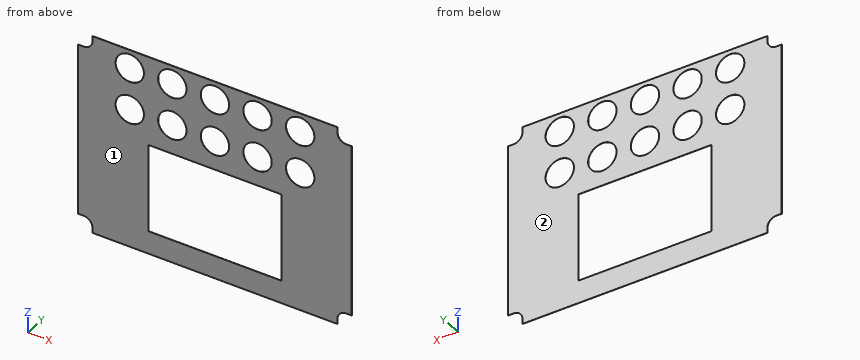
from build123d import *

# Parameters (mm, degrees)
SKETCH1_W           = 154
SKETCH1_H           = 114
BOSS_EXTRUDE1_DEPTH = 0.1
CUT_EXTRUDE1_DEPTH  = 3
SKETCH3_R           = 8
SKETCH3_W           = 75
SKETCH3_H           = 50
CUT_EXTRUDE2_DEPTH  = 1


with BuildPart() as part:
    # Sketch1 → Boss-Extrude1 (new body)
    with BuildSketch(Plane(origin=(0, 0, 0), x_dir=(1, 0, 0), z_dir=(0, 1, 0))):
        Rectangle(SKETCH1_W, SKETCH1_H)
    extrude(amount=BOSS_EXTRUDE1_DEPTH)

    # Sketch2 → Cut-Extrude1 (cut)
    with BuildSketch(Plane(origin=(0, 0.1, 0), x_dir=(1, 0, 0), z_dir=(0, 1, 0))):
        with BuildLine():
            Line((-52.05, -19.483379374), (-52.05, -25.516620626))
            ThreePointArc((-52.05, -25.516620626), (-48, -27.55), (-43.95, -25.516620626))
            Line((-43.95, -25.516620626), (-43.95, -19.483379374))
            ThreePointArc((-43.95, -19.483379374), (-48, -17.45), (-52.05, -19.483379374))
        make_face()
        with BuildLine():
            Line((-19.95, -19.483379374), (-19.95, -25.516620626))
            ThreePointArc((-19.95, -25.516620626), (-24, -27.55), (-28.05, -25.516620626))
            Line((-28.05, -25.516620626), (-28.05, -19.483379374))
            ThreePointArc((-28.05, -19.483379374), (-24, -17.45), (-19.95, -19.483379374))
        make_face()
        with BuildLine():
            Line((4.05, -19.483379374), (4.05, -25.516620626))
            ThreePointArc((4.05, -25.516620626), (0, -27.55), (-4.05, -25.516620626))
            Line((-4.05, -25.516620626), (-4.05, -19.483379374))
            ThreePointArc((-4.05, -19.483379374), (0, -17.45), (4.05, -19.483379374))
        make_face()
        with BuildLine():
            Line((28.05, -19.483379374), (28.05, -25.516620626))
            ThreePointArc((28.05, -25.516620626), (24, -27.55), (19.95, -25.516620626))
            Line((19.95, -25.516620626), (19.95, -19.483379374))
            ThreePointArc((19.95, -19.483379374), (24, -17.45), (28.05, -19.483379374))
        make_face()
        with BuildLine():
            Line((52.05, -19.483379374), (52.05, -25.516620626))
            ThreePointArc((52.05, -25.516620626), (48, -27.55), (43.95, -25.516620626))
            Line((43.95, -25.516620626), (43.95, -19.483379374))
            ThreePointArc((43.95, -19.483379374), (48, -17.45), (52.05, -19.483379374))
        make_face()
        with BuildLine():
            Line((-19.95, -43.483379374), (-19.95, -49.516620626))
            ThreePointArc((-19.95, -49.516620626), (-24, -51.55), (-28.05, -49.516620626))
            Line((-28.05, -49.516620626), (-28.05, -43.483379374))
            ThreePointArc((-28.05, -43.483379374), (-24, -41.45), (-19.95, -43.483379374))
        make_face()
        with BuildLine():
            Line((4.05, -43.483379374), (4.05, -49.516620626))
            ThreePointArc((4.05, -49.516620626), (0, -51.55), (-4.05, -49.516620626))
            Line((-4.05, -49.516620626), (-4.05, -43.483379374))
            ThreePointArc((-4.05, -43.483379374), (0, -41.45), (4.05, -43.483379374))
        make_face()
        with BuildLine():
            Line((28.05, -43.483379374), (28.05, -49.516620626))
            ThreePointArc((28.05, -49.516620626), (24, -51.55), (19.95, -49.516620626))
            Line((19.95, -49.516620626), (19.95, -43.483379374))
            ThreePointArc((19.95, -43.483379374), (24, -41.45), (28.05, -43.483379374))
        make_face()
        with BuildLine():
            Line((52.05, -43.483379374), (52.05, -49.516620626))
            ThreePointArc((52.05, -49.516620626), (48, -51.55), (43.95, -49.516620626))
            Line((43.95, -49.516620626), (43.95, -43.483379374))
            ThreePointArc((43.95, -43.483379374), (48, -41.45), (52.05, -43.483379374))
        make_face()
        with BuildLine():
            Line((-43.95, -43.483379374), (-43.95, -49.516620626))
            ThreePointArc((-43.95, -49.516620626), (-48, -51.55), (-52.05, -49.516620626))
            Line((-52.05, -49.516620626), (-52.05, -43.483379374))
            ThreePointArc((-52.05, -43.483379374), (-48, -41.45), (-43.95, -43.483379374))
        make_face()
    extrude(amount=-CUT_EXTRUDE1_DEPTH, mode=Mode.SUBTRACT)

    # Sketch3 → Cut-Extrude2 (cut)
    # profile 1 of 15: a face of its own
    with BuildSketch(Plane(origin=(0, 0.1, 0), x_dir=(1, 0, 0), z_dir=(0, 1, 0))):
        with BuildLine():
            Line((-69, 57), (-77, 57))
            Line((-77, 57), (-77, 49))
            Line((-77, 49), (-74, 49))
            ThreePointArc((-74, 49), (-70.464466094, 50.464466094), (-69, 54))
            Line((-69, 54), (-69, 57))
        make_face()
    # profile 2 of 15: a face of its own
    with BuildSketch(Plane(origin=(0, 0.1, 0), x_dir=(1, 0, 0), z_dir=(0, 1, 0))):
        with BuildLine():
            Line((77, 57), (69, 57))
            Line((69, 57), (69, 54))
            ThreePointArc((69, 54), (70.464466094, 50.464466094), (74, 49))
            Line((74, 49), (77, 49))
            Line((77, 49), (77, 57))
        make_face()
    # profile 3 of 15: a face of its own
    with BuildSketch(Plane(origin=(0, 0.1, 0), x_dir=(1, 0, 0), z_dir=(0, 1, 0))):
        with BuildLine():
            Line((77, -57), (77, -49))
            Line((77, -49), (74, -49))
            ThreePointArc((74, -49), (70.464466094, -50.464466094), (69, -54))
            Line((69, -54), (69, -57))
            Line((69, -57), (77, -57))
        make_face()
    # profile 4 of 15: a face of its own
    with BuildSketch(Plane(origin=(0, 0.1, 0), x_dir=(1, 0, 0), z_dir=(0, 1, 0))):
        with BuildLine():
            Line((-74, -49), (-77, -49))
            Line((-77, -49), (-77, -57))
            Line((-77, -57), (-69, -57))
            Line((-69, -57), (-69, -54))
            ThreePointArc((-69, -54), (-70.464466094, -50.464466094), (-74, -49))
        make_face()
    # profile 5 of 15: a face of its own
    with BuildSketch(Plane(origin=(0, 0.1, 0), x_dir=(1, 0, 0), z_dir=(0, 1, 0))):
        with Locations(Location((-48, -22.5, 0), (0, 0, 270))):
            Circle(SKETCH3_R)
        with BuildLine():
            Line((-52.05, -25.516620626), (-52.05, -19.483379374))
            ThreePointArc((-52.05, -19.483379374), (-48, -17.45), (-43.95, -19.483379374))
            Line((-43.95, -19.483379374), (-43.95, -25.516620626))
            ThreePointArc((-43.95, -25.516620626), (-48, -27.55), (-52.05, -25.516620626))
        make_face(mode=Mode.SUBTRACT)
    # profile 6 of 15: a face of its own
    with BuildSketch(Plane(origin=(0, 0.1, 0), x_dir=(1, 0, 0), z_dir=(0, 1, 0))):
        with Locations(Location((-24, -22.5, 0), (0, 0, 270))):
            Circle(SKETCH3_R)
        with BuildLine():
            Line((-28.05, -25.516620626), (-28.05, -19.483379374))
            ThreePointArc((-28.05, -19.483379374), (-24, -17.45), (-19.95, -19.483379374))
            Line((-19.95, -19.483379374), (-19.95, -25.516620626))
            ThreePointArc((-19.95, -25.516620626), (-24, -27.55), (-28.05, -25.516620626))
        make_face(mode=Mode.SUBTRACT)
    # profile 7 of 15: a face of its own
    with BuildSketch(Plane(origin=(0, 0.1, 0), x_dir=(1, 0, 0), z_dir=(0, 1, 0))):
        with Locations(Location((0, -22.5, 0), (0, 0, 270))):
            Circle(SKETCH3_R)
        with BuildLine():
            Line((-4.05, -25.516620626), (-4.05, -19.483379374))
            ThreePointArc((-4.05, -19.483379374), (0, -17.45), (4.05, -19.483379374))
            Line((4.05, -19.483379374), (4.05, -25.516620626))
            ThreePointArc((4.05, -25.516620626), (0, -27.55), (-4.05, -25.516620626))
        make_face(mode=Mode.SUBTRACT)
    # profile 8 of 15: a face of its own
    with BuildSketch(Plane(origin=(0, 0.1, 0), x_dir=(1, 0, 0), z_dir=(0, 1, 0))):
        with Locations(Location((24, -22.5, 0), (0, 0, 270))):
            Circle(SKETCH3_R)
        with BuildLine():
            Line((19.95, -25.516620626), (19.95, -19.483379374))
            ThreePointArc((19.95, -19.483379374), (24, -17.45), (28.05, -19.483379374))
            Line((28.05, -19.483379374), (28.05, -25.516620626))
            ThreePointArc((28.05, -25.516620626), (24, -27.55), (19.95, -25.516620626))
        make_face(mode=Mode.SUBTRACT)
    # profile 9 of 15: a face of its own
    with BuildSketch(Plane(origin=(0, 0.1, 0), x_dir=(1, 0, 0), z_dir=(0, 1, 0))):
        with Locations(Location((48, -22.5, 0), (0, 0, 270))):
            Circle(SKETCH3_R)
        with BuildLine():
            Line((43.95, -25.516620626), (43.95, -19.483379374))
            ThreePointArc((43.95, -19.483379374), (48, -17.45), (52.05, -19.483379374))
            Line((52.05, -19.483379374), (52.05, -25.516620626))
            ThreePointArc((52.05, -25.516620626), (48, -27.55), (43.95, -25.516620626))
        make_face(mode=Mode.SUBTRACT)
    # profile 10 of 15: a face of its own
    with BuildSketch(Plane(origin=(0, 0.1, 0), x_dir=(1, 0, 0), z_dir=(0, 1, 0))):
        with Locations(Location((48, -46.5, 0), (0, 0, 270))):
            Circle(SKETCH3_R)
        with BuildLine():
            Line((43.95, -49.516620626), (43.95, -43.483379374))
            ThreePointArc((43.95, -43.483379374), (48, -41.45), (52.05, -43.483379374))
            Line((52.05, -43.483379374), (52.05, -49.516620626))
            ThreePointArc((52.05, -49.516620626), (48, -51.55), (43.95, -49.516620626))
        make_face(mode=Mode.SUBTRACT)
    # profile 11 of 15: a face of its own
    with BuildSketch(Plane(origin=(0, 0.1, 0), x_dir=(1, 0, 0), z_dir=(0, 1, 0))):
        with Locations(Location((24, -46.5, 0), (0, 0, 270))):
            Circle(SKETCH3_R)
        with BuildLine():
            Line((19.95, -49.516620626), (19.95, -43.483379374))
            ThreePointArc((19.95, -43.483379374), (24, -41.45), (28.05, -43.483379374))
            Line((28.05, -43.483379374), (28.05, -49.516620626))
            ThreePointArc((28.05, -49.516620626), (24, -51.55), (19.95, -49.516620626))
        make_face(mode=Mode.SUBTRACT)
    # profile 12 of 15: a face of its own
    with BuildSketch(Plane(origin=(0, 0.1, 0), x_dir=(1, 0, 0), z_dir=(0, 1, 0))):
        with Locations(Location((0, -46.5, 0), (0, 0, 270))):
            Circle(SKETCH3_R)
        with BuildLine():
            Line((-4.05, -49.516620626), (-4.05, -43.483379374))
            ThreePointArc((-4.05, -43.483379374), (0, -41.45), (4.05, -43.483379374))
            Line((4.05, -43.483379374), (4.05, -49.516620626))
            ThreePointArc((4.05, -49.516620626), (0, -51.55), (-4.05, -49.516620626))
        make_face(mode=Mode.SUBTRACT)
    # profile 13 of 15: a face of its own
    with BuildSketch(Plane(origin=(0, 0.1, 0), x_dir=(1, 0, 0), z_dir=(0, 1, 0))):
        with Locations(Location((-24, -46.5, 0), (0, 0, 270))):
            Circle(SKETCH3_R)
        with BuildLine():
            Line((-28.05, -49.516620626), (-28.05, -43.483379374))
            ThreePointArc((-28.05, -43.483379374), (-24, -41.45), (-19.95, -43.483379374))
            Line((-19.95, -43.483379374), (-19.95, -49.516620626))
            ThreePointArc((-19.95, -49.516620626), (-24, -51.55), (-28.05, -49.516620626))
        make_face(mode=Mode.SUBTRACT)
    # profile 14 of 15: a face of its own
    with BuildSketch(Plane(origin=(0, 0.1, 0), x_dir=(1, 0, 0), z_dir=(0, 1, 0))):
        with Locations(Location((-48, -46.5, 0), (0, 0, 270))):
            Circle(SKETCH3_R)
        with BuildLine():
            Line((-52.05, -49.516620626), (-52.05, -43.483379374))
            ThreePointArc((-52.05, -43.483379374), (-48, -41.45), (-43.95, -43.483379374))
            Line((-43.95, -43.483379374), (-43.95, -49.516620626))
            ThreePointArc((-43.95, -49.516620626), (-48, -51.55), (-52.05, -49.516620626))
        make_face(mode=Mode.SUBTRACT)
    # profile 15 of 15: a face of its own
    with BuildSketch(Plane(origin=(0, 0.1, 0), x_dir=(1, 0, 0), z_dir=(0, 1, 0))):
        with Locations((0, 19)):
            Rectangle(SKETCH3_W, SKETCH3_H)
    extrude(amount=-CUT_EXTRUDE2_DEPTH, mode=Mode.SUBTRACT)


solid = part.part
Work out the finished part from the listing and answer in its coordinate system (mm). Face numbers are marked on the shaded views. Round coordinates to 2 decimals unless told otherwise and drop trailing zeros. Write each loop counter-clockwise with the first axis right and the second up, starting at its lowest first coordinate (ties: lowest second). Pieces come first, ordered by that corner, then holes. Notation, with made-up numbers: (86.5, -8.75) -> (120.5, -8.75) arc R28 ccw to (120.5, 26.25) -> close; hole circle Ø5 at (13, 71). An arc over 180 degrees is marked (long way). Answer as CSV lines item,"result". Start each with the question number.
(1) This flat-tipped pin is pushed along its axis until it touches: pin 1 (14.5 mm diameter, centred on x = 0, z = 22.5, fed in from +Y). Where does it stop, or does it pass through?
(2) The mould has two halves that part along Y. Classify the marked faces 1 and 2: +Y half, -Y half, draft (parallel to the pull), parting line (faces both ways), or undercut.
(3) Find the intervals of material crossed by probe 1 along X at (y, z) = (0.05, 46.5); probe 2 along X at (y, z) = (0.05, -9), in increasing order.
(4) The part is cut by section D-D, the plane z = -1.5. Give the vertices of the cut face in (x, y).
(5) The part is cut by section A-A, the plane z = 46.5. Give the vertices of the cut face in (x, y).
(6) The part is cut by section B-B, the plane x = 48. Give the vertices of the cut face in (y, z).
(7) The part is cut by section C-C, the plane x = 24. Give the vertices of the cut face in (y, z).
Output values:
1,pin 1,"passes through"
2,face 1,"-Y half"
2,face 2,"+Y half"
3,probe 1,"x = -77 to -56, -40 to -32, -16 to -8, 8 to 16, 32 to 40, 56 to 77"
3,probe 2,"x = -77 to -37.5, 37.5 to 77"
4,outline,"(-77, 0) -> (-37.5, 0) -> (-37.5, 0.1) -> (-77, 0.1) -> close; (37.5, 0) -> (77, 0) -> (77, 0.1) -> (37.5, 0.1) -> close"
5,outline,"(-77, 0) -> (-56, 0) -> (-56, 0.1) -> (-77, 0.1) -> close; (-40, 0) -> (-32, 0) -> (-32, 0.1) -> (-40, 0.1) -> close; (-16, 0) -> (-8, 0) -> (-8, 0.1) -> (-16, 0.1) -> close; (8, 0) -> (16, 0) -> (16, 0.1) -> (8, 0.1) -> close; (32, 0) -> (40, 0) -> (40, 0.1) -> (32, 0.1) -> close; (56, 0) -> (77, 0) -> (77, 0.1) -> (56, 0.1) -> close"
6,outline,"(0, -57) -> (0.1, -57) -> (0.1, 14.5) -> (0, 14.5) -> close; (0, 30.5) -> (0.1, 30.5) -> (0.1, 38.5) -> (0, 38.5) -> close; (0, 54.5) -> (0.1, 54.5) -> (0.1, 57) -> (0, 57) -> close"
7,outline,"(0, -57) -> (0.1, -57) -> (0.1, -44) -> (0, -44) -> close; (0, 6) -> (0.1, 6) -> (0.1, 14.5) -> (0, 14.5) -> close; (0, 30.5) -> (0.1, 30.5) -> (0.1, 38.5) -> (0, 38.5) -> close; (0, 54.5) -> (0.1, 54.5) -> (0.1, 57) -> (0, 57) -> close"
